Design review of the part built by this model. Coordinates are the model's own, in mm. Face numbers are marked on the shaded views. A direction names the side the tool comes from. Coordinates: 2 decimals unless noted, no trailing zeros. Loops run counter-clockwise (first coordinate to the right, second up) from the corner with the lowest first, then second, coordinate; pieces in that order, holes last.
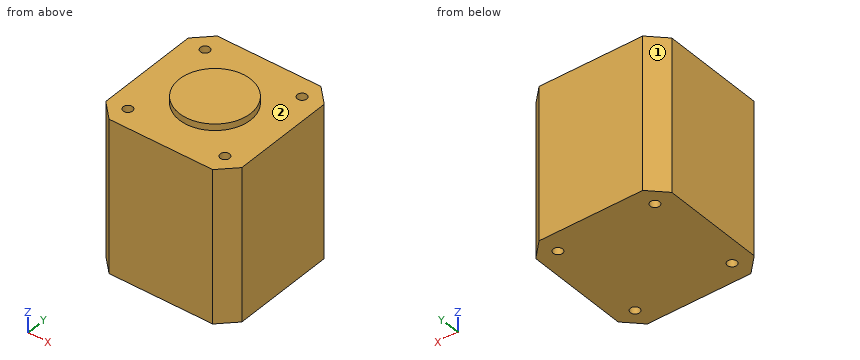
from build123d import *

# Parameters (mm, degrees)
F0_W     = 42
F0_H     = 42
F1_DEPTH = 47.15
F2_SIZE  = 5
F3_R     = 1.44
F4_DEPTH = 47.15
F5_R     = 10.99
F6_DEPTH = 2


with BuildPart() as f1:
    # F0 (on Top) → F1 (new body)
    with BuildSketch(Plane.XY):
        Rectangle(F0_W, F0_H)
    extrude(amount=F1_DEPTH)

    # F2
    f2_edges = [f1.edges().sort_by_distance(p)[0] for p in [
        (-21, 21, 23.575),
        (-21, -21, 23.575),
        (21, -21, 23.575),
        (21, 21, 23.575),
    ]]
    chamfer(f2_edges, length=F2_SIZE)

    # F3 (on face) → F4 (cut, through all)
    with BuildSketch(Plane.XY.offset(47.15)):
        with Locations((14.97, 14.973074)):
            Circle(F3_R)
        with Locations((14.97, -14.973074)):
            Circle(F3_R)
        with Locations((-14.97, -14.973074)):
            Circle(F3_R)
        with Locations((-14.97, 14.973074)):
            Circle(F3_R)
    extrude(amount=-F4_DEPTH, mode=Mode.SUBTRACT)

    # F5 (on face) → F6 (join)
    with BuildSketch(Plane.XY.offset(47.15)):
        Circle(F5_R)
    extrude(amount=F6_DEPTH)


solid = f1.part
Q1. Take a section at A-A, the plane x = -14.97. Write out the cut boundary in (y, z), then the cut area to 3 significant figures.
Q2. For line 1 (Y direction, x = -14.97, z = 14); line 2 (Z direction, x = -15.5, y = 16.5); line 3 (X direction, y = 16, z = 42.5), list the stretches that pass through material, from the lowest coordinate up.
Q3. Take a section at D-D, the plane y = 4.5. Write out the cut boundary in (x, z), then the cut area to 3 significant figures.
Q4. Take a section at B-B, the plane z = 45.5. Write out the cut boundary in (x, y), then the cut area to 3 significant figures.
Q5. Take a section at C-C, the plane x = 0. Write out the cut boundary in (y, z).
Q6. Machinability: for the marked faces 1 and 2, which of the approach directions +Z, -Z, +X, -X, +Y, -Y give a long, thin tool a straight path to every point of the face, cutting with its end or side? Answer none if there is none.
Q7. Clearance check with a flat-ended pin moving along its axis: pin 1 Ø4.5 at (x, y) = (14.97, 14.97) entering from +Z. State where the tip first meets the part, or that it passes through.
Entries:
1. outline: (-21, 0) - (-16.41, 0) - (-16.41, 47.15) - (-21, 47.15) - close; (-13.53, 0) - (13.53, 0) - (13.53, 47.15) - (-13.53, 47.15) - close; (16.41, 0) - (21, 0) - (21, 47.15) - (16.41, 47.15) - close
1. area: 1,710 mm2
2. line 1: y = -21 to -16.41, -13.53 to 13.53, 16.41 to 21
2. line 2: z = 0 to 47.15
2. line 3: x = -21 to -15.98, -13.96 to 13.96, 15.98 to 21
3. outline: (-21, 0) - (21, 0) - (21, 47.15) - (10.03, 47.15) - (10.03, 49.15) - (-10.03, 49.15) - (-10.03, 47.15) - (-21, 47.15) - close
3. area: 2,020 mm2
4. outline: (-21, -16) - (-16, -21) - (16, -21) - (21, -16) - (21, 16) - (16, 21) - (-16, 21) - (-21, 16) - close; hole circle Ø2.88 at (-14.97, -14.97); hole circle Ø2.88 at (-14.97, 14.97); hole circle Ø2.88 at (14.97, -14.97); hole circle Ø2.88 at (14.97, 14.97)
4. area: 1,690 mm2
5. outline: (-21, 0) - (21, 0) - (21, 47.15) - (10.99, 47.15) - (10.99, 49.15) - (-10.99, 49.15) - (-10.99, 47.15) - (-21, 47.15) - close
6. face 1: +Z, -Z, -X, +Y
6. face 2: +Z
7. pin 1: stops at z = 47.15
